Geometry: see drawing. Coordinates: mm, zero at the bounding-box minimum. A direction names the side the tool comes from. Coordinates: 2 decimals unless noted, no trailing zeros. Write each loop counter-clockwise with the first axis right and the second up, starting at its lowest first coordinate (ties: lowest second). Pieces come first, ordered by that corner, then holes.
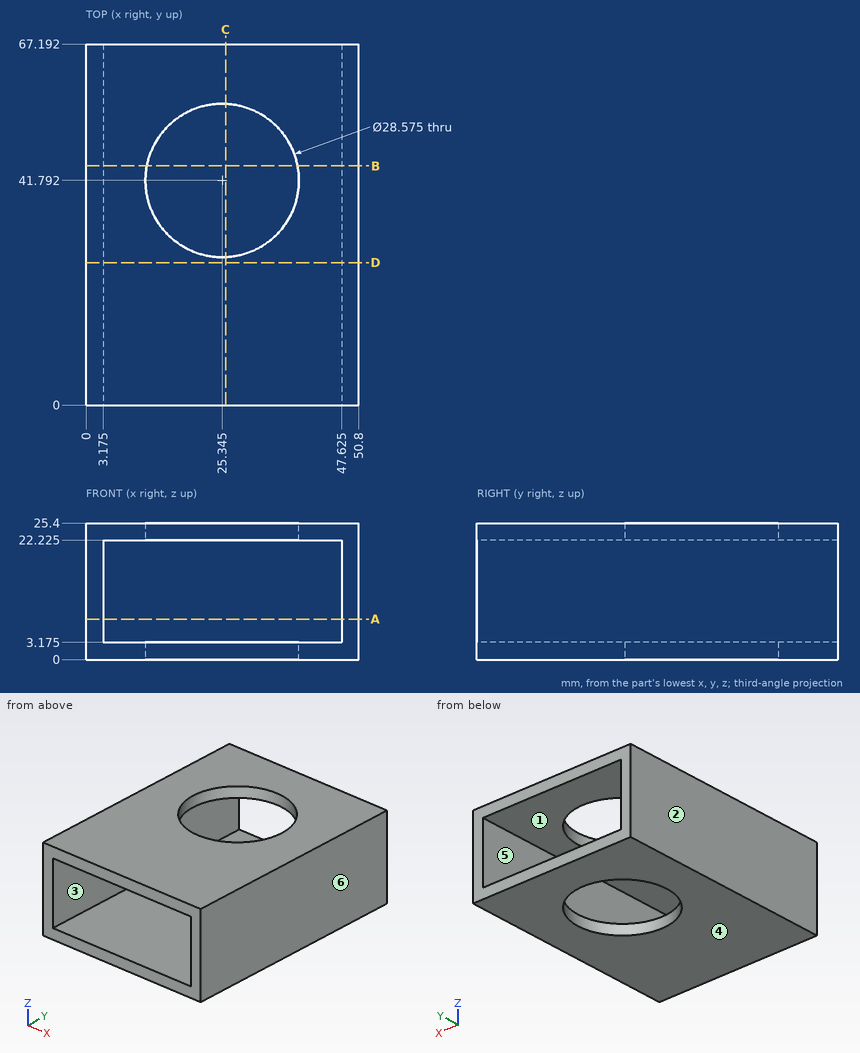
Item 1: Set-up query: the marked faces 1 and 2. Return all of +Z, -Z, +X, -X, +Y, -Y with unobstructed straight access to the full face (end or side cutting, diameter ignored); none if empty.
Derived:
face 1: +Y, -Y
face 2: +Z, -Z, -X, +Y, -Y
Item 2: Pin query (flat end, axial travel): pin 1 (5 mm diameter, centred on x = 42.5, z = 21, fed in from -Y); pin 2 (23 mm diameter, centred on x = 25.35, y = 41.79, fed in from +Z). Return the tip coordinate at first contact, or that it passes through.
Derived:
pin 1: stops at y = 0
pin 2: passes through
Item 3: Section B-B, the plane y = 44.5. Output: boundary loops of the cut face in (x, z) (1 decimal).
Derived:
outline: (0, 0) - (11.3, 0) - (11.3, 3.2) - (3.2, 3.2) - (3.2, 22.2) - (11.3, 22.2) - (11.3, 25.4) - (0, 25.4) - close; (39.4, 0) - (50.8, 0) - (50.8, 25.4) - (39.4, 25.4) - (39.4, 22.2) - (47.6, 22.2) - (47.6, 3.2) - (39.4, 3.2) - close
Item 4: Section D-D, the plane y = 26.5. Output: boundary loops of the cut face in (x, z) (1 decimal).
Derived:
outline: (0, 0) - (50.8, 0) - (50.8, 25.4) - (0, 25.4) - close; hole (3.2, 3.2) - (47.6, 3.2) - (47.6, 22.2) - (3.2, 22.2) - close
Item 5: Section A-A, the plane z = 7.5. Output: boundary loops of the cut face in (x, y) (1 decimal).
Derived:
outline: (0, 0) - (3.2, 0) - (3.2, 67.2) - (0, 67.2) - close; (47.6, 0) - (50.8, 0) - (50.8, 67.2) - (47.6, 67.2) - close
Item 6: Section C-C, the plane x = 26. Output: boundary loops of the cut face in (y, z) (1 decimal).
Derived:
outline: (0, 0) - (27.5, 0) - (27.5, 3.2) - (0, 3.2) - close; (0, 22.2) - (27.5, 22.2) - (27.5, 25.4) - (0, 25.4) - close; (56.1, 0) - (67.2, 0) - (67.2, 3.2) - (56.1, 3.2) - close; (56.1, 22.2) - (67.2, 22.2) - (67.2, 25.4) - (56.1, 25.4) - close
Item 7: Pull-direction query (Z, two-part tool) for the marked faces 3, 4, 5 and 6; classes: released by +Z, released by -Z, zero draft, split by the parting line, or undercut.
Derived:
face 3: undercut
face 4: released by -Z
face 5: undercut
face 6: zero draft
Item 8: Material intervals for probe 1 along X at (y, z) = (60.5, 17.5) (1 decimal); probe 2 along Z at (x, y) = (46.5, 19.5) (1 decimal); probe 3 along Y at (x, z) = (25.5, 2.25) (1 decimal), sorted ascending.
Derived:
probe 1: x = 0 to 3.2, 47.6 to 50.8
probe 2: z = 0 to 3.2, 22.2 to 25.4
probe 3: y = 0 to 27.5, 56.1 to 67.2
